CAD build for the part. Positions are in the model's coordinates, mm. Round coordinates to 2 decimals unless told otherwise and drop trailing zeros. Loops run counter-clockwise (first coordinate to the right, second up) from the corner with the lowest first, then second, coordinate; pieces in that order, holes last. Notation, with made-up numbers: M 30,84.5 L 69,84.5 A33 cw 69,118.5 Z; hole C 29,10.25 d10. An arc over 180 degrees is marked long. Put each result on its own line as item: value. Start each with the question number.
from build123d import *

# Parameters (mm, degrees)
SKETCH_1_W                 = 153.4
SKETCH_1_H                 = 10
EXTRUDE_1_DEPTH            = 3
CUT_EXTRUDE_1_DEPTH        = 78.407299397
PATTERN_LINEAR_1_COUNT     = 21
PATTERN_LINEAR_1_PITCH     = 6.28
PATTERN_LINEAR_1_COL_COUNT = 2
PATTERN_LINEAR_1_COL_PITCH = 6.28
SKETCH_3_W                 = 10
SKETCH_3_H                 = 3
CUT_EXTRUDE_2_DEPTH        = 78.407299397
SKETCH_4_W                 = 5
SKETCH_4_H                 = 3
EXTRUDE_2_DEPTH            = 38.5
EXTRUDE_START              = -5
EXTRUDE_1_2_OUTLINE_W      = 10
EXTRUDE_1_2_OUTLINE_H      = 25
EXTRUDE_1_2_DEPTH          = 5
SKETCH_6_R                 = 2
CUT_EXTRUDE_3_DEPTH        = 6
CUT_EXTRUDE_START          = -6
SKETCH_7_R                 = 2
CUT_EXTRUDE_4_DEPTH        = 6


# Read off the part's stored shape, not the designer's step: 돌출-얇게1
with BuildPart() as part:
    # 스케치1 → Extrude 1 (new body)
    with BuildSketch(Plane.XY):
        with Locations((0, 5)):
            Rectangle(SKETCH_1_W, SKETCH_1_H)
    extrude(amount=-EXTRUDE_1_DEPTH)

    # 스케치2 → 컷-돌출1 (cut, through all)
    with BuildSketch(Plane.XY):
        Polygon((-67.94, 8), (-67.94, 10), (-70.237940469, 10), (-69.51, 8), align=None)
        Polygon((-65.642059531, 10), (-67.94, 10), (-67.94, 8), (-66.37, 8), align=None)
        Polygon((-66.37, 8), (-67.94, 8), (-67.94, 5.5), (-67.279925586, 5.5), align=None)
        Polygon((-67.94, 5.5), (-67.94, 8), (-69.51, 8), (-68.600074414, 5.5), align=None)
    cut_extrude_1 = extrude(amount=-CUT_EXTRUDE_1_DEPTH, mode=Mode.SUBTRACT)

    # 선형 패턴1: 컷-돌출1 ×21
    with Locations(*[(i * PATTERN_LINEAR_1_PITCH, 0, 0) for i in range(1, PATTERN_LINEAR_1_COUNT)]):
        add(cut_extrude_1, mode=Mode.SUBTRACT)

    # 선형 패턴1 col: 컷-돌출1 ×2
    with Locations(*[(-i * PATTERN_LINEAR_1_COL_PITCH, 0, 0) for i in range(1, PATTERN_LINEAR_1_COL_COUNT)]):
        add(cut_extrude_1, mode=Mode.SUBTRACT)

    # 스케치3 → 컷-돌출2 (cut, through all)
    with BuildSketch(Plane.XZ):
        with Locations((71.7, -1.5)):
            Rectangle(SKETCH_3_W, SKETCH_3_H)
    extrude(amount=-CUT_EXTRUDE_2_DEPTH, mode=Mode.SUBTRACT)

    # 스케치4 → 보스-돌출2 (add)
    with BuildSketch(Plane(origin=(0, 0, 0), x_dir=(-1, 0, 0), z_dir=(0, -1, 0))):
        with Locations((-64.2, 1.5)):
            Rectangle(SKETCH_4_W, SKETCH_4_H)
    extrude(amount=EXTRUDE_2_DEPTH)

    # Extrude 1 2 outline → Extrude 1 2 (add)
    with BuildSketch(Plane.XY.offset(EXTRUDE_START)):
        with Locations((71.7, -26)):
            Rectangle(EXTRUDE_1_2_OUTLINE_W, EXTRUDE_1_2_OUTLINE_H)
    extrude(amount=EXTRUDE_1_2_DEPTH)

    # 스케치6 → 컷-돌출3 (cut)
    with BuildSketch(Plane(origin=(0, -38.5, 0), x_dir=(-1, 0, 0), z_dir=(0, -1, 0))):
        with Locations(Location((-71.7, 2.5, 0), (0, 0, 90))):
            Circle(SKETCH_6_R)
    extrude(amount=-CUT_EXTRUDE_3_DEPTH, mode=Mode.SUBTRACT)

    # 스케치7 → 컷-돌출4 (cut)
    with BuildSketch(Plane(origin=(0, -13.5, 0), x_dir=(1, 0, 0), z_dir=(0, 1, 0)).offset(CUT_EXTRUDE_START)):
        with Locations(Location((71.7, 2.5, 0), (0, 0, 90))):
            Circle(SKETCH_7_R)
    extrude(amount=CUT_EXTRUDE_4_DEPTH, mode=Mode.SUBTRACT)


solid = part.part
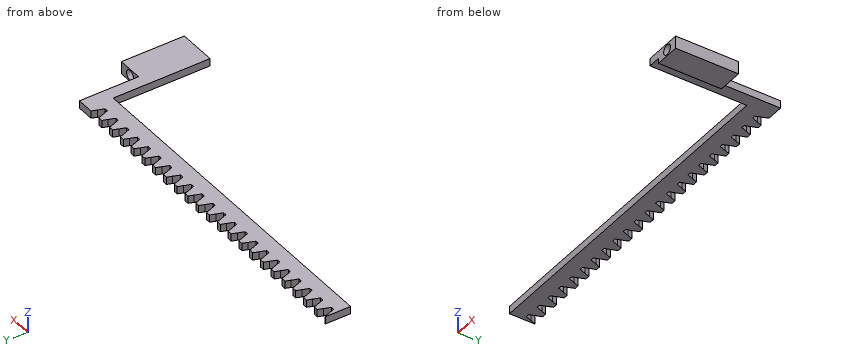
(1) Flat gauge pins, fed straight in: pin 1 Ø1.2 at (x, z) = (71.5, -3) entering from -Y; pin 2 Ø2 at (y, z) = (-11, -1.5) entering from +X; pin 3 Ø1.5 at (x, z) = (25.5, -1) entering from -Y. Where does each tip first touch, or does it go through?
(2) Cut at A-A on x = 71.7. List the corners of the cut face in (y, z), and give its area (3 significant figures).
(3) Cut at B-B on y = -27.5. List the corners of the cut face in (x, z).
(4) Cut at C-C on y = -6. List the corners of the cut face in (x, z).
(5) Drill centre lines: line 1 along X through (y, z) = (-16.75, -2.5); line 2 along Z through (x, y) = (71.7, -17.55); line 3 along Z through (x, y) = (71, -35). Where is each one in solid material? Low to high.
Taken from the geometry:
1. pin 1: y = -32.5
1. pin 2: x = 66.7
1. pin 3: y = 0
2. outline: M -38.5,-5 L -13.5,-5 L -13.5,-4.5 L -19.5,-4.5 L -19.5,-0.5 L -13.5,-0.5 L -13.5,0 L -38.5,0 L -38.5,-0.5 L -32.5,-0.5 L -32.5,-4.5 L -38.5,-4.5 Z
2. area: 77.0 mm2
3. outline: M 61.7,-3 L 66.7,-3 L 66.7,-5 L 76.7,-5 L 76.7,0 L 61.7,0 Z
4. outline: M 61.7,-3 L 66.7,-3 L 66.7,0 L 61.7,0 Z
5. line 1: 61.7 to 69.7, 73.7 to 76.7
5. line 2: -5 to -4.5, -0.5 to 0
5. line 3: -5 to -4.37, -0.63 to 0
